```python
from build123d import *

# Parameters (mm, degrees)
SKETCH1_R                = 3
BOSS_EXTRUDE4_DEPTH      = 5
SKETCH4_W                = 5.761442696
SKETCH4_H                = 28
BOSS_EXTRUDE5_DEPTH      = 47
SKETCH6_W                = 5.761442696
SKETCH6_H                = 28
SKETCH6_R                = 14
SKETCH6_R_2              = 3
BOSS_EXTRUDE6_DEPTH      = 5
SKETCH8_R                = 8
SKETCH8_R_2              = 3.1
BOSS_EXTRUDE7_DEPTH      = 17.61
BOSS_EXTRUDE7_DEPTH_BACK = 74.61
BOSS_EXTRUDE8_DEPTH      = 57
FILLET1_R                = 10
FILLET2_R                = 10
CUT_EXTRUDE1_DEPTH       = 57
SKETCH14_R               = 1.395
CUT_EXTRUDE2_DEPTH       = 3


with BuildPart() as part:
    # Sketch1 → Boss-Extrude4 (new body)
    with BuildSketch(Plane(origin=(0, 0, 0), x_dir=(1, 0, 0), z_dir=(0, 1, 0))):
        with BuildLine():
            Line((-62.942048288, -14), (-22.942048288, -14))
            ThreePointArc((-22.942048288, -14), (-8.942048288, 0), (-22.942048288, 14))
            Line((-22.942048288, 14), (-62.942048288, 14))
            Line((-62.942048288, 14), (-62.942048288, -14))
        make_face()
        with Locations((-22.942048288, 0)):
            Circle(SKETCH1_R, mode=Mode.SUBTRACT)
    extrude(amount=BOSS_EXTRUDE4_DEPTH)

    # Sketch4 → Boss-Extrude5 (add)
    with BuildSketch(Plane(origin=(0, 5, 0), x_dir=(1, 0, 0), z_dir=(0, 1, 0))):
        with Locations((-60.06132694, 0)):
            Rectangle(SKETCH4_W, SKETCH4_H)
    extrude(amount=BOSS_EXTRUDE5_DEPTH)

    # Sketch6 → Boss-Extrude6 (add)
    with BuildSketch(Plane(origin=(0, 52, 0), x_dir=(1, 0, 0), z_dir=(0, 1, 0))):
        with BuildLine():
            ThreePointArc((-22.942048288, -14), (-36.942048288, 0), (-22.942048288, 14))
            Line((-22.942048288, 14), (-57.180605592, 14))
            Line((-57.180605592, 14), (-57.180605592, -14))
            Line((-57.180605592, -14), (-22.942048288, -14))
        make_face()
        with Locations((-60.06132694, 0)):
            Rectangle(SKETCH6_W, SKETCH6_H)
        with Locations((-22.942048288, 0)):
            Circle(SKETCH6_R)
        with Locations((-22.942048288, 0)):
            Circle(SKETCH6_R_2, mode=Mode.SUBTRACT)
    extrude(amount=BOSS_EXTRUDE6_DEPTH)



with BuildPart() as body_2:
    # Sketch8 → Boss-Extrude7 (new body, two sides)
    with BuildSketch(Plane(origin=(0, 57, 0), x_dir=(1, 0, 0), z_dir=(0, 1, 0))) as boss_extrude7_sk:
        with Locations((-74.942048288, 0)):
            Circle(SKETCH8_R)
        with Locations((-74.942048288, 0)):
            Circle(SKETCH8_R_2, mode=Mode.SUBTRACT)
    extrude(amount=BOSS_EXTRUDE7_DEPTH)
    extrude(boss_extrude7_sk.sketch, amount=-BOSS_EXTRUDE7_DEPTH_BACK)


with BuildPart() as part_1:
    add(part.part)

    add(body_2.part)  # Boss-Extrude8 merges body 2
    # Sketch11 → Boss-Extrude8 (add)
    with BuildSketch(Plane.XZ):
        with BuildLine():
            Line((-62.942048288, 14), (-74.942048288, 8))
            ThreePointArc((-74.942048288, 8), (-69.285194038, 5.656854249), (-66.942048288, 0))
            ThreePointArc((-66.942048288, 0), (-69.285194038, -5.656854249), (-74.942048288, -8))
            Line((-74.942048288, -8), (-62.942048288, -14))
            Line((-62.942048288, -14), (-62.942048288, 14))
        make_face()
    extrude(amount=-BOSS_EXTRUDE8_DEPTH)

    # Fillet1
    fillet1_edges = [part_1.edges().sort_by_distance(p)[0] for p in [
        (-62.942048288, 28.5, 14),
        (-62.942048288, 28.5, -14),
    ]]
    fillet(fillet1_edges, radius=FILLET1_R)

    # Fillet2
    fillet2_edges = [part_1.edges().sort_by_distance(p)[0] for p in [
        (-74.942048288, 28.5, 8),
        (-74.942048288, 28.5, -8),
    ]]
    fillet(fillet2_edges, radius=FILLET2_R)

    # Sketch13 → Cut-Extrude1 (cut)
    with BuildSketch(Plane.XZ):
        with BuildLine():
            Line((-60.581368513, 6), (-39.338409666, 6))
            ThreePointArc((-39.338409666, 6), (-33.338409666, 0), (-39.338409666, -6))
            Line((-39.338409666, -6), (-60.581368513, -6))
            ThreePointArc((-60.581368513, -6), (-66.581368513, 0), (-60.581368513, 6))
        make_face()
    extrude(amount=-CUT_EXTRUDE1_DEPTH, mode=Mode.SUBTRACT)

    # Sketch14 → Cut-Extrude2 (cut)
    with BuildSketch(Plane(origin=(0, 57, 0), x_dir=(1, 0, 0), z_dir=(0, 1, 0))):
        with Locations((-22.942048288, 7.4422)):
            Circle(SKETCH14_R)
        with Locations((-22.942048288, -7.4422)):
            Circle(SKETCH14_R)
    extrude(amount=-CUT_EXTRUDE2_DEPTH, mode=Mode.SUBTRACT)


solid = part_1.part
```
Work out the finished part from the listing and answer in its coordinate system (mm). A direction names the side the tool comes from. Round coordinates to 2 decimals unless told otherwise and drop trailing zeros. Loops run counter-clockwise (first coordinate to the right, second up) from the corner with the lowest first, then second, coordinate; pieces in that order, holes last. Notation, with made-up numbers: M 71.5,10.25 L 95.5,10.25 A15 ccw 95.5,26.25 Z; hole C -36,82 d8. An arc over 180 degrees is marked long. One line per question, with ' | ' between items.
Q1. Consider line 1 along X through (y, z) = (54.8, 0); line 2 along Y through (x, z) = (-49.5, 7.25); line 3 along Z through (x, y) = (-50, 1). Determine where each line is inside the solid, lowest interval first. Write a range as from..to.
Conclusion:
line 1: x = -82.94..-78.04, -71.84..-66.58, -33.34..-25.94, -19.94..-8.94 | line 2: y = 0..5, 52..57 | line 3: z = -14..-6, 6..14
Q2. Find section A-A, the plane x = -40.5. Give the vertices of the cut face in (y, z).
Conclusion:
outline: M 0,-14 L 5,-14 L 5,-6 L 0,-6 Z; M 0,6 L 5,6 L 5,14 L 0,14 Z; M 52,-14 L 57,-14 L 57,-6 L 52,-6 Z; M 52,6 L 57,6 L 57,14 L 52,14 Z
Q3. Each of these flat-tipped pins is pushed along its axis until it touches: pin 1 Ø0.8 at (x, z) = (-23, -7) entering from +Y; pin 2 Ø2.5 at (x, z) = (-22.94, -7.44) entering from -Y; pin 3 Ø8 at (y, z) = (63.5, -7.5) entering from +X; pin 4 Ø5 at (y, z) = (21.5, 1.5) entering from -X. Where does it stop, or does it pass through?
Conclusion:
pin 1: stops at y = 54 | pin 2: stops at y = 0 | pin 3: stops at x = -67.75 | pin 4: stops at x = -82.94
Q4. Find section C-C, the plane y = 1.5. Give the vertices of the cut face in (x, z), then the cut area to 3 significant figures.
Conclusion:
outline: M -76.19,-7.9 A10 cw -73.27,-8.84 L -65.05,-12.94 A10 ccw -60.58,-14 L -22.94,-14 A14 ccw -22.94,14 L -60.58,14 A10 ccw -65.05,12.94 L -73.27,8.84 A10 cw -76.19,7.9 A8 ccw Z; hole C -74.94,0 d6.2; hole M -60.58,-6 L -39.34,-6 A6 ccw -39.34,6 L -60.58,6 A6 ccw Z; hole C -22.94,0 d6 | area: 1,370 mm2
Q5. Find section B-B, the plane z = 0. Give the vertices of the cut face in (x, y), then the cut area to 3 significant figures.
Conclusion:
outline: M -82.94,-17.61 L -78.04,-17.61 L -78.04,74.61 L -82.94,74.61 Z; M -71.84,-17.61 L -66.94,-17.61 L -66.94,0 L -66.58,0 L -66.58,57 L -66.94,57 L -66.94,74.61 L -71.84,74.61 Z; M -33.34,0 L -25.94,0 L -25.94,5 L -33.34,5 Z; M -33.34,52 L -25.94,52 L -25.94,57 L -33.34,57 Z; M -19.94,0 L -8.94,0 L -8.94,5 L -19.94,5 Z; M -19.94,52 L -8.94,52 L -8.94,57 L -19.94,57 Z | area: 1,110 mm2
Q6. A tool of negligible diameter and unlimited length cuts with its end or side. For faces 1 (the flat face through (-33, 5, -3)), 2 (the cylindrical face through (-81.29, 29.15, 4.87)), 3 (the flat face through (-60, 28, 6)), 4 (the cylindrical face through (-24.336, 55.521, -7.504)), from which of +Z, -Z, +X, -X, +Y, -Y can it reach the whole face along a straight path? Write none if from no direction.
Conclusion:
face 1: +Z, -Z, +X | face 2: none | face 3: +Y, -Y | face 4: +Y
Q7. The mould has two halves that part along X. Classify faces 5 (the flat face through (-57.181, 28, 10)), 6 (the flat face through (-58, 28, -6)), 7 (the cylindrical face through (-74.71, 28.9, -8.25)): +X half, -X half, draft (parallel to the pull), parting line (faces both ways), or undercut.
Conclusion:
face 5: +X half | face 6: undercut | face 7: -X half
Q8. Find section D-D, the plane x = -64. Give the vertices of the cut face in (y, z).
Conclusion:
outline: M 0,-13.4 L 57,-13.4 L 57,-4.93 L 0,-4.93 Z; M 0,4.93 L 57,4.93 L 57,13.4 L 0,13.4 Z
